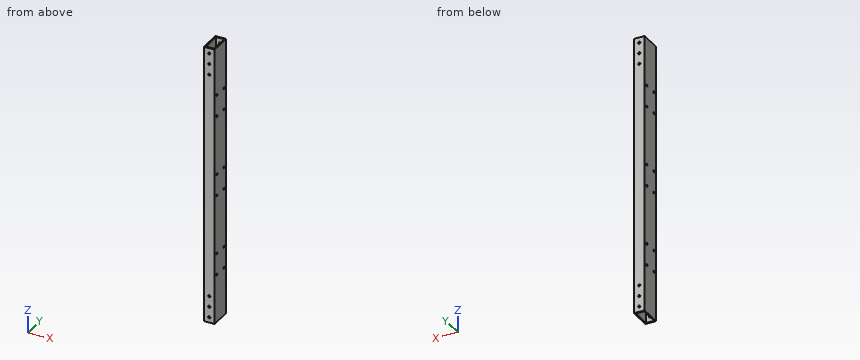
Autodesk Inventor part; units mm, degrees
ref_plane "YZ Plane" through (0, 0, 0) normal (1, 0, 0) x (0, 1, 0)
ref_plane "XZ Plane" through (0, 0, 0) normal (0, 1, 0) x (-1, 0, 0)
ref_plane "XY Plane" through (0, 0, 0) normal (0, 0, 1) x (1, 0, 0)
sketch "Sketch1" plane through (0, 0, 0) normal (0, 0, 1) x (1, 0, 0)
  line L0 (0, 0) -> (25.4, 0)
  line L1 (25.4, 0) -> (25.4, 50.8)
  line L2 (25.4, 50.8) -> (0, 50.8)
  line L3 (0, 50.8) -> (0, 0)
  line L4 (3.175, 3.175) -> (22.225, 3.175)
  line L5 (22.225, 3.175) -> (22.225, 47.625)
  line L6 (22.225, 47.625) -> (3.175, 47.625)
  line L7 (3.175, 47.625) -> (3.175, 3.175)
  dimension "d0" = 25.4
  dimension "d1" = 50.8
  dimension "d2" = 3.175
  dimension "d3" = 3.175
  dimension "d4" = 3.175
  dimension "d5" = 3.175
extrude "Extrusion1" add sketch "Sketch1" along normal blind 660.4
sketch "Sketch2" plane through (0, 50.8, 0) normal (0, 1, 0) x (1, 0, 0)
  line L0 (25.4, 0) -> (0, 0)
  line L1 (12.7, 0) -> (12.7, -660.4)
  line L2 (0, -660.4) -> (25.4, -660.4)
  line L3 (12.7, -660.4) -> (12.7, -647.7)
  line L4 (12.7, -647.7) -> (12.7, -622.3)
  line L5 (12.7, -622.3) -> (12.7, -596.9)
  circle A0 centre (12.7, -647.7) radius 2.54
  circle A1 centre (12.7, -622.3) radius 2.54
  circle A2 centre (12.7, -596.9) radius 2.54
  line L6 (12.7, 0) -> (12.7, -12.7)
  line L7 (12.7, -12.7) -> (12.7, -38.1)
  line L8 (12.7, -38.1) -> (12.7, -63.5)
  circle A3 centre (12.7, -63.5) radius 2.54
  circle A4 centre (12.7, -38.1) radius 2.54
  circle A5 centre (12.7, -12.7) radius 2.54
  dimension "d8" = 12.7
  dimension "d9" = 25.4
  dimension "d10" = 25.4
  dimension "d11" = 5.08
  dimension "d12" = 12.7
  dimension "d13" = 25.4
  dimension "d14" = 25.4
extrude "Extrusion2" cut sketch "Sketch2" against normal blind 660.4
sketch "Sketch3" plane through (25.4, 0, 0) normal (1, 0, 0) x (0, 0, -1)
  line L0 (0, 50.8) -> (-660.4, 50.8)
  line L1 (0, 50.8) -> (-114.3, 50.8)
  line L2 (-114.3, 50.8) -> (-165.1, 50.8)
  line L3 (-114.3, 50.8) -> (-114.3, 41.275)
  line L4 (-165.1, 50.8) -> (-165.1, 41.275)
  circle A0 centre (-165.1, 41.275) radius 2.54
  circle A1 centre (-114.3, 41.275) radius 2.54
  line L5 (-165.1, 0) -> (-165.1, 9.525)
  line L6 (0, 0) -> (-660.4, 0)
  line L7 (-114.3, 0) -> (-114.3, 9.525)
  circle A2 centre (-165.1, 9.525) radius 2.54
  circle A3 centre (-114.3, 9.525) radius 2.54
  dimension "d17" = 114.3
  dimension "d18" = 50.8
  dimension "d19" = 9.525
  dimension "d20" = 5.08
  dimension "d21" = 9.525
extrude "Extrusion3" cut sketch "Sketch3" against normal blind 660.4
sketch "Sketch4" plane through (25.4, 0, 0) normal (1, 0, 0) x (0, 0, -1)
  circle A0 centre (-165.1, 41.275) radius 2.54
  line L0 (-165.1, 41.275) -> (-304.8, 41.275)
  line L1 (-304.8, 41.275) -> (-355.6, 41.275)
  line L2 (-355.6, 41.275) -> (-355.6, 9.525)
  line L3 (-355.6, 9.525) -> (-304.8, 9.525)
  circle A1 centre (-304.8, 41.275) radius 2.54
  circle A2 centre (-355.6, 41.275) radius 2.54
  circle A3 centre (-355.6, 9.525) radius 2.54
  circle A4 centre (-304.8, 9.525) radius 2.54
  point P0 (0, 0)
  dimension "d24" = 139.7
  dimension "d25" = 50.8
extrude "Extrusion4" cut sketch "Sketch4" against normal blind 660.4 contours A4 | A3 L3 L2 | L2 L3 A3 | A2 L2 L1 | L1 L2 A2 | A1 L1 L0 | L0 L1 A1
sketch "Sketch5" plane through (25.4, 0, 0) normal (1, 0, 0) x (0, 0, -1)
  circle A0 centre (-355.6, 41.275) radius 2.54
  line L0 (-355.6, 41.275) -> (-495.3, 41.275)
  line L1 (-495.3, 41.275) -> (-546.1, 41.275)
  line L2 (-546.1, 41.275) -> (-546.1, 9.525)
  line L3 (-546.1, 9.525) -> (-495.3, 9.525)
  circle A1 centre (-495.3, 41.275) radius 2.54
  circle A2 centre (-546.1, 41.275) radius 2.54
  circle A3 centre (-546.1, 9.525) radius 2.54
  circle A4 centre (-495.3, 9.525) radius 2.54
  point P0 (0, 0)
  dimension "d28" = 139.7
  dimension "d29" = 50.8
extrude "Extrusion5" cut sketch "Sketch5" against normal blind 660.4 contours A4 | A3 L3 L2 | L2 L3 A3 | A2 L2 L1 | L1 L2 A2 | A1 L1 L0 | L0 L1 A1
properties part number "26 1x2" material "Aluminum 6061"
Part model, mm, in its own coordinate system. Round coordinates to 2 decimals unless told otherwise and drop trailing zeros. Write each loop counter-clockwise with the first axis right and the second up, starting at its lowest first coordinate (ties: lowest second). Pieces come first, ordered by that corner, then holes. Notation, with made-up numbers: (-2, -12.75) -> (11, -12.75) arc R15 cw to (11, -5.75) -> close; hole circle Ø4 at (-6.75, -20). An arc over 180 degrees is marked (long way). Return JSON: item names as keys, results as strings. Group by question number.
Q1. Saw through at A-A on y = 19.5. Write the cut outline in (x, z) (3 decimals).
Q2. Saw through at B-B on z = 223.5. Write the cut outline in (x, y) (3 decimals).
Q3. Probe L1, parallel to Y at x = 1.45, z = 355.6 (3 decimals); L2, parallel to X at y = 12, z = 493.5 (3 decimals); L3, parallel to Y at x = 14.25, z = 164 (3 decimals). List the from-to ranges inside material, lowest first. Write a range as [from, to].
Q4. Pin check, flat tip, straight feed: pin 1 (4 mm diameter, centred on y = 9.525, z = 495.3, fed in from -X). Stop position of the tip, or through.
Answer:
{
 "1": {"outline": "(0, 0) -> (3.175, 0) -> (3.175, 660.4) -> (0, 660.4) -> close; (22.225, 0) -> (25.4, 0) -> (25.4, 660.4) -> (22.225, 660.4) -> close"},
 "2": {"outline": "(0, 0) -> (25.4, 0) -> (25.4, 50.8) -> (0, 50.8) -> close; hole (3.175, 3.175) -> (22.225, 3.175) -> (22.225, 47.625) -> (3.175, 47.625) -> close"},
 "3": {"L1": "[0, 6.985], [12.065, 38.735], [43.815, 50.8]", "L2": "[0, 3.175], [22.225, 25.4]", "L3": "[0, 3.175], [47.625, 50.8]"},
 "4": {"pin 1": "through"}
}
